For this review, use the dimensioned drawing (mm, ordinates from the lowest corner) and the shaded views. Coordinates: 2 decimals unless noted, no trailing zeros. Order: outer loops, then holes, each group sorted by start corner. A loop starts at its lowest first (then second) coordinate and runs counter-clockwise, first axis right, second up. Notation, with made-up numbers: M 40.5,-16.75 L 69.5,-16.75 A21 ccw 69.5,11.25 Z; hole C 79.5,73 d10. An arc over 180 degrees is marked long. Answer in a Markdown table with one row per item.
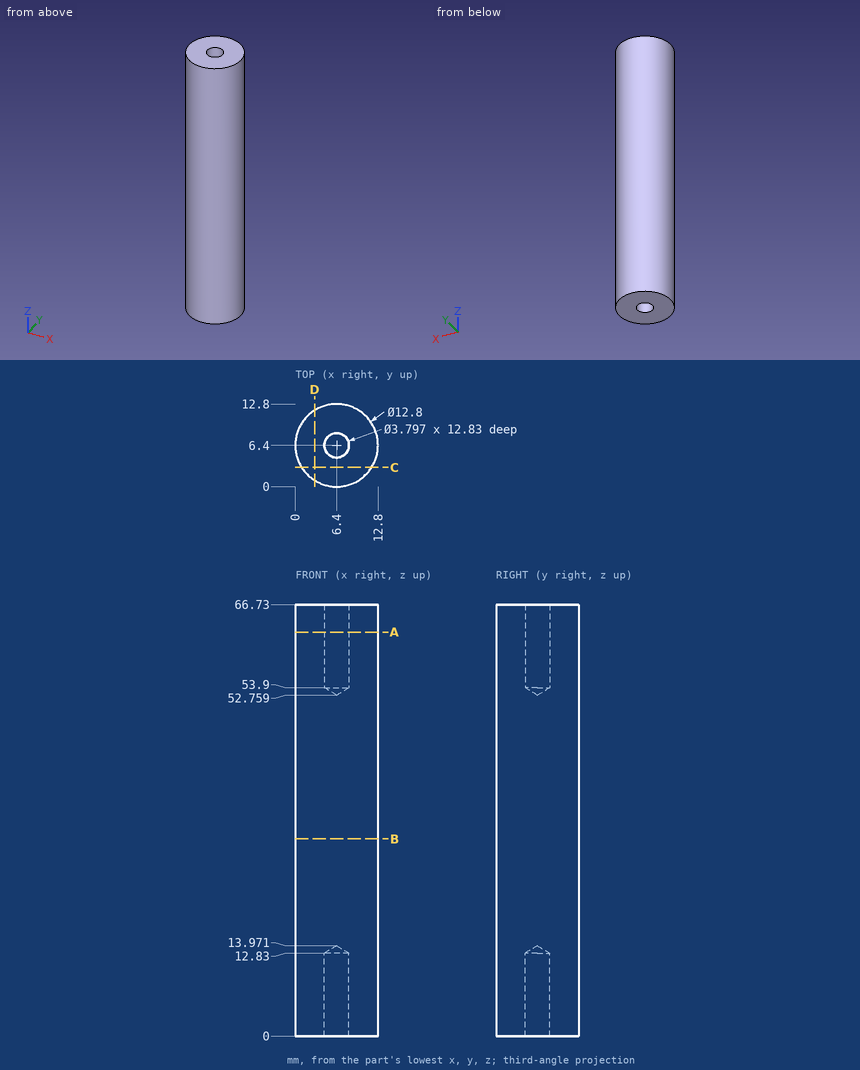
(1) To check wall thickness, follow line 1 (Y direction, x = 6.4, z = 6.5); line 2 (Y direction, x = 7.5, z = 61.5) (1 decimal). State the ranges of each line that lie inside material, in increasing order. Write a range as [from, to].
Report:
| item | result |
|---|---|
| line 1 | [0, 4.5], [8.3, 12.8] |
| line 2 | [0.1, 4.9], [7.9, 12.7] |
(2) Insertion check: P1, Ø3.5, axis at x = 6.4, y = 6.4, coming from the +Z side; P2, Ø3, axis at x = 9, z = 45, coming from the +Y side (1 decimal); P3, Ø2, axis at y = 1.5, z = 57, coming from the +X side (1 decimal). Each pin has a flat end and moves straight along its axis. Give the tip position at first contact, or say it passes through.
Report:
| item | result |
|---|---|
| P1 | z = 53.81 |
| P2 | y = 12.7 |
| P3 | x = 11.5 |
(3) Take a section at A-A (z = 62.5). Write out the cut boundary in (x, y).
Report:
| item | result |
|---|---|
| outline | C 6.4,6.4 d12.8; hole C 6.4,6.4 d3.8 |
(4) Take a section at B-B (z = 30.5). Write out the cut boundary in (x, y).
Report:
| item | result |
|---|---|
| outline | C 6.4,6.4 d12.8 |
(5) Take a section at C-C (y = 3). Write out the cut boundary in (x, z), then the cut area to 3 significant figures.
Report:
| item | result |
|---|---|
| outline | M 0.98,0 L 11.82,0 L 11.82,66.73 L 0.98,66.73 Z |
| area | 724 mm^2 |
